Input: part model. Units: mm. Frame: model coordinates. Face numbers are marked on the shaded views. A direction names the side the tool comes from. Round coordinates to 2 decimals unless told otherwise and drop trailing zeros. Loops run counter-clockwise (first coordinate to the right, second up) from the corner with the lowest first, then second, coordinate; pieces in that order, holes last.
1) First-contact query: pin 1 (4 mm diameter, centred on x = 6, z = -3.5, fed in from +Y); pin 2 (6 mm diameter, centred on x = -4, y = 5.5, fed in from -Z); pin 3 (2 mm diameter, centred on x = 4.5, z = 37, fed in from +Y); pin 4 (10 mm diameter, centred on x = 0, z = 41.5, fed in from -Y) (3 decimals). Flat tips, straight axial feed; report the tip coordinate or a pass-through.
2) Access query for the marked faces 1, 2 and 3. Directions: +Z, -Z, +X, -X, +Y, -Y. A direction counts if a zero-diameter tool reaches every point of the face in a straight line with its end or side. Return the directions, or none.
3) Section A-A, the plane x = 0. Return loops of the section in (y, z) (3 decimals).
4) Section D-D, the plane y = 5.5. Return loops of the section in (x, z).
5) Section C-C, the plane z = 27.5. Return loops of the section in (x, y).
6) Ray query, line 1 along Z through (x, y) = (-6.25, -4.5); line 2 along Z through (x, y) = (4.75, -0.5); line 3 along X through (y, z) = (-0.25, 1). Return the intervals inside material, ascending.
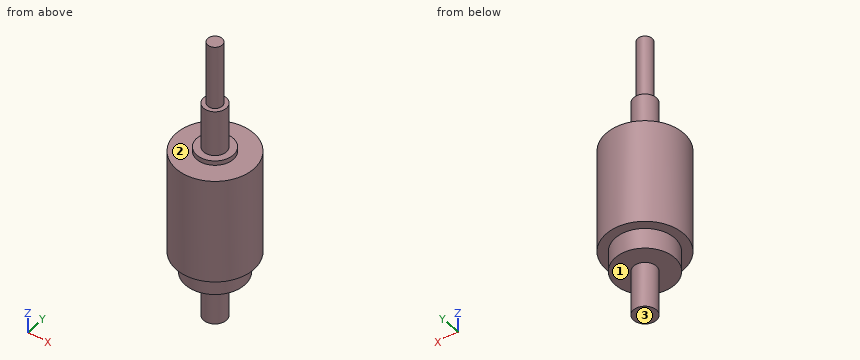
from build123d import *

# Parameters (mm, degrees)
SKETCH1_R           = 8.5
BOSS_EXTRUDE1_DEPTH = 23
SKETCH2_R           = 4
BOSS_EXTRUDE2_DEPTH = 1
SKETCH3_R           = 2.5
BOSS_EXTRUDE3_DEPTH = 10
SKETCH4_R           = 6.5
BOSS_EXTRUDE4_DEPTH = 4.5
BOSS_EXTRUDE5_START = 10
SKETCH5_R           = 2.5
BOSS_EXTRUDE5_DEPTH = 10
SKETCH7_R           = 1.585
BOSS_EXTRUDE6_DEPTH = 14


with BuildPart() as part:
    # Sketch1 → Boss-Extrude1 (new body)
    with BuildSketch(Plane.XY):
        Circle(SKETCH1_R)
    extrude(amount=BOSS_EXTRUDE1_DEPTH)

    # Sketch2 → Boss-Extrude2 (add)
    with BuildSketch(Plane.XY.offset(23)):
        Circle(SKETCH2_R)
    extrude(amount=BOSS_EXTRUDE2_DEPTH)

    # Sketch3 → Boss-Extrude3 (add)
    with BuildSketch(Plane.XY.offset(24)):
        Circle(SKETCH3_R)
    extrude(amount=BOSS_EXTRUDE3_DEPTH)

    # Sketch4 → Boss-Extrude4 (add)
    with BuildSketch(Plane(origin=(0, 0, 0), x_dir=(-1, 0, 0), z_dir=(0, 0, -1))):
        Circle(SKETCH4_R)
    extrude(amount=BOSS_EXTRUDE4_DEPTH)

    # Sketch5 → Boss-Extrude5 (add)
    with BuildSketch(Plane(origin=(0, 0, -4.5), x_dir=(-1, 0, 0), z_dir=(0, 0, -1)).offset(BOSS_EXTRUDE5_START)):
        with Locations(Location((0, 0, 0), (0, 0, 180))):
            Circle(SKETCH5_R)
    extrude(amount=-BOSS_EXTRUDE5_DEPTH)

    # Sketch7 → Boss-Extrude6 (add)
    with BuildSketch(Plane.XY.offset(34)):
        Circle(SKETCH7_R)
    extrude(amount=BOSS_EXTRUDE6_DEPTH)


solid = part.part
Final values:
1. pin 1: stops at y = 5.12
1. pin 2: stops at z = -4.5
1. pin 3: passes through
1. pin 4: stops at y = -1.585
2. face 1: -Z
2. face 2: +Z
2. face 3: -Z, +X, -X, +Y, -Y
3. outline: (-8.5, 0) - (-6.5, 0) - (-6.5, -4.5) - (-2.5, -4.5) - (-2.5, -14.5) - (2.5, -14.5) - (2.5, -4.5) - (6.5, -4.5) - (6.5, 0) - (8.5, 0) - (8.5, 23) - (4, 23) - (4, 24) - (2.5, 24) - (2.5, 34) - (1.585, 34) - (1.585, 48) - (-1.585, 48) - (-1.585, 34) - (-2.5, 34) - (-2.5, 24) - (-4, 24) - (-4, 23) - (-8.5, 23) - close
4. outline: (-6.48, 0) - (-3.46, 0) - (-3.46, -4.5) - (3.46, -4.5) - (3.46, 0) - (6.48, 0) - (6.48, 23) - (-6.48, 23) - close
5. outline: circle Ø5 at (0, 0)
6. line 1: z = 0 to 23
6. line 2: z = -4.5 to 23
6. line 3: x = -8.5 to 8.5
